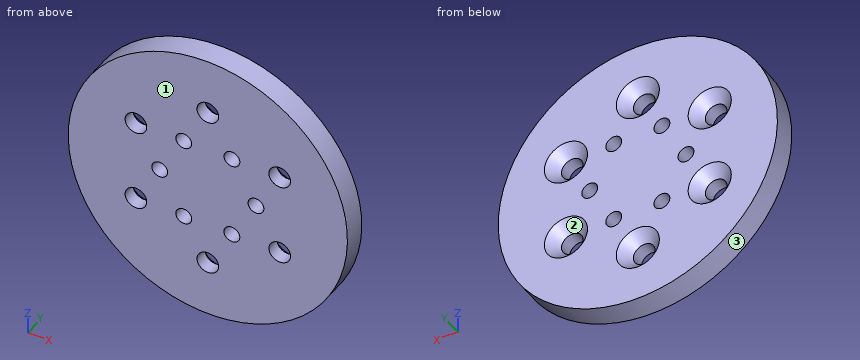
```python
from build123d import *

# Parameters (mm, degrees)
SKIZZE1_R                                            = 29
AUFSATZ_LINEAR_AUSTRAGEN1_DEPTH                      = 5
FORMSENKUNG_F_R_M4_SENKSCHRAUBE_MIT_INNE_D           = 4.5
FORMSENKUNG_F_R_M4_SENKSCHRAUBE_MIT_INNE_CSINK_D     = 8.96
FORMSENKUNG_F_R_M4_SENKSCHRAUBE_MIT_INNE_CSINK_ANGLE = 90
M4_GEWINDEBOHRUNG1_D                                 = 3.3


with BuildPart() as part:
    # Skizze1 → Aufsatz-Linear austragen1 (new body)
    with BuildSketch(Plane(origin=(0, 0, 0), x_dir=(1, 0, 0), z_dir=(0, 1, 0))):
        with Locations(Location((0, 0, 0), (0, 0, 270))):
            Circle(SKIZZE1_R)
    extrude(amount=AUFSATZ_LINEAR_AUSTRAGEN1_DEPTH)

    # Formsenkung für M4 Senkschraube mit Innensechskant1 (through all)
    with Locations(Plane(origin=(0, 5, 0), x_dir=(1, 0, 0), z_dir=(0, 1, 0))):
        with Locations((-14.938938215, 8.625), (0, 17.25), (14.938938215, 8.625), (14.938938215, -8.625), (0, -17.25), (-14.938938215, -8.625)):
            CounterSinkHole(FORMSENKUNG_F_R_M4_SENKSCHRAUBE_MIT_INNE_D / 2, FORMSENKUNG_F_R_M4_SENKSCHRAUBE_MIT_INNE_CSINK_D / 2, counter_sink_angle=FORMSENKUNG_F_R_M4_SENKSCHRAUBE_MIT_INNE_CSINK_ANGLE)

    # M4 Gewindebohrung1 (through all)
    with Locations(Plane(origin=(0, 5, 0), x_dir=(1, 0, 0), z_dir=(0, 1, 0))):
        with Locations((-10, 0), (-5, 8.660254038), (5, 8.660254038), (10, 0), (5, -8.660254038), (-5, -8.660254038)):
            Hole(M4_GEWINDEBOHRUNG1_D / 2)


solid = part.part
```
Could you check a few things on this model? Use its own coordinates, in mm. Face numbers are marked on the shaded views. Coordinates: 2 decimals unless noted, no trailing zeros. Write each loop counter-clockwise with the first axis right and the second up, starting at its lowest first coordinate (ties: lowest second). Pieces come first, ordered by that corner, then holes. Notation, with made-up numbers: (11.25, 77.5) -> (27.25, 77.5) arc R23 ccw to (27.25, 96.5) -> close; hole circle Ø2 at (59.25, -21). An arc over 180 degrees is marked (long way). Write item = value, one per line. Start each with the question number.
(1) I want a section at C-C (x = 25). Please give me the cut outline in (y, z), plus the area to 3 significant figures.
(2) I need wall thicknesses on line 1 (Z direction, x = -2, y = 4); line 2 (Z direction, x = 15.5, y = 2.65); line 3 (X direction, y = 0.65, z = 8). Which ranges of each line are inside material? Lowest first, please. Write a range as [from, to].
(3) We'd pull the mould along Z, two halves only. Please class the marked faces 1, 2 and 3: released by +Z, released by -Z, zero draft, split by the parting line, or undercut.
(4) I want a section at A-A (y = 1.5). Give the number of separate pieces and of enclosed holes in the cut face, plus the area to 3 significant figures.
(5) Will these pins go through, and if not, where does the flat tip stop? pin 1 (5.5 mm diameter, centred on x = -10, z = 0, fed in from +Y); pin 2 (7 mm diameter, centred on x = 14.94, z = -8.62, fed in from +Y); pin 3 (3.5 mm diameter, centred on x = 0, z = -17.25, fed in from -Y); pin 4 (3 mm diameter, centred on x = -8, y = 4.5, fed in from +Z).
Result set:
q1.outline = (0, -14.7) -> (5, -14.7) -> (5, 14.7) -> (0, 14.7) -> close
q1.area = 147 mm2
q2.line_1 = [-28.93, -20.1], [-14.4, 14.4], [20.1, 28.93]
q2.line_2 = [-24.51, -10.8], [-6.45, 6.45], [10.8, 24.51]
q2.line_3 = [-27.87, -17.1], [-12.78, -6.51], [-3.49, 3.49], [6.51, 12.78], [17.1, 27.87]
q3.face_1 = zero draft
q3.face_2 = undercut
q3.face_3 = split by the parting line
q4.separate_pieces = 1
q4.enclosed_holes = 12
q4.area = 2,500 mm2
q5.pin_1 = 5
q5.pin_2 = 4.03
q5.pin_3 = through
q5.pin_4 = 28.26
